The listing builds one solid part. Answer for the finished solid, in the listing's coordinates (mm). A direction names the side the tool comes from. Round coordinates to 2 decimals unless told otherwise and drop trailing zeros. Order: outer loops, then holes, each group sorted by start corner. A loop starts at its lowest first (then second) coordinate and runs counter-clockwise, first axis right, second up. Notation, with made-up numbers: (46.5, 51.25) - (105.5, 51.25) arc R26 cw to (105.5, 86.25) - close; hole circle Ø8 at (-7.75, -31.5). An arc over 180 degrees is marked (long way). One line per item, written item: value. Start each with the question number.
1. Section B-B, the plane z = -0.3 is taken. Give the vertices of the cut face in (x, y).
2. Section A-A, the plane y = -0.25 is taken. Give the vertices of the cut face in (x, z).
3. For a pull along X with two mould halves and no side action, classify faces 1 (the flat face through (3, 2, 0)), 2 (the flat face through (6.1, -3, -1.5)), 3 (the flat face through (3, 0, -2)), 4 (the flat face through (6.4, 0.5, -1.5)) as released by +X, released by -X, zero draft, split by the parting line, or undercut.
4. Section D-D, the plane y = 3.75 is taken. Give the vertices of the cut face in (x, z).
5. Flat-ended cylindrical pins translate along their axes: P1, Ø0.6, axis at y = 4, z = -1.5, coming from the +X side; P2, Ø0.5, axis at y = -3, z = -1.5, coming from the +X side; P3, Ø0.5, axis at y = -3, z = -1.5, coming from the -X side; P4, Ø2, axis at x = 1, y = -1.5, coming from the -Z side. Find the tip coordinate at first contact, or state that the pin passes through.
6. Section C-C, the plane x = 0.5 is taken. Give the vertices of the cut face in (y, z), then the cut area to 3 significant figures.
7. Straight lines are drawn through the part: line 1 (Y direction, x = 1.25, z = -2.8); line 2 (X direction, y = 3.25, z = -0.6); line 3 (X direction, y = -2.25, z = -1.75). For each, find the intervals that lie inside material, in ascending order.
8. A tool of negligible diameter and unlimited length cuts with its end or side. For faces 5 (the flat face through (3, 4.3, -2)), 6 (the flat face through (-0.4, 0.5, -1.5)), from which of +Z, -Z, +X, -X, +Y, -Y can it reach the whole face along a straight path? Write none if from no direction.
from build123d import *

# Parameters (mm, degrees)
SKETCH1_W           = 6
SKETCH1_H           = 3
BOSS_EXTRUDE1_DEPTH = 3.5
BOSS_EXTRUDE2_DEPTH = 0.5
SKETCH3_W           = 3
SKETCH3_H           = 1.5
BOSS_EXTRUDE3_DEPTH = 0.8
FILLET1_R           = 0.05


with BuildPart() as part:
    # Sketch1 → Boss-Extrude1 (new body)
    with BuildSketch(Plane(origin=(0, 0, 0), x_dir=(1, 0, 0), z_dir=(0, 1, 0))):
        with Locations((3, 1.5)):
            Rectangle(SKETCH1_W, SKETCH1_H)
    extrude(amount=BOSS_EXTRUDE1_DEPTH)

    # Sketch2 → Boss-Extrude2 (add, symmetric)
    with BuildSketch(Plane.XY.offset(-1.5)):
        Polygon((-0.1, 1.7), (0, 1.7), (0, 2), (-0.4, 2), (-0.4, -0.925735931), (-1.224264069, -1.75), (-0.4, -2.574264069), (-0.4, -3.5), (-0.1, -3.5), (-0.1, -2.45), (-0.8, -1.75), (-0.1, -1.05), (-0.1, -0.722730952), align=None)
    boss_extrude2 = extrude(amount=BOSS_EXTRUDE2_DEPTH, both=True)

    # Mirror1: Boss-Extrude2 across plane
    add(boss_extrude2.mirror(Plane.ZY.offset(-3)))

    # Sketch3 → Boss-Extrude3 (add)
    with BuildSketch(Plane(origin=(0, 3.5, 0), x_dir=(1, 0, 0), z_dir=(0, 1, 0))):
        with Locations((3, 1.5)):
            Rectangle(SKETCH3_W, SKETCH3_H)
    extrude(amount=BOSS_EXTRUDE3_DEPTH)

    # Fillet1
    fillet1_edges = [part.edges().sort_by_distance(p)[0] for p in [
        (6, 3.5, -1.5),
        (3, 3.5, -3),
        (-0.4, -3.5, -1.5),
        (-0.4, -3.037132034, -2),
        (-0.4, -2.574264069, -1.5),
        (-0.812132034, -2.162132034, -2),
        (-1.224264069, -1.75, -1.5),
        (-0.812132034, -1.337867966, -2),
        (-0.4, -0.925735931, -1.5),
        (-0.4, 0.537132034, -2),
        (-0.4, 2, -1.5),
        (0, 2, -1.5),
        (0, 1.85, -1),
        (0, 1.7, -1.5),
        (0, 1.85, -2),
        (-0.45, -2.1, -2),
        (-0.4, -3.037132034, -1),
        (-0.4, 0.537132034, -1),
        (-0.812132034, -1.337867966, -1),
        (-0.812132034, -2.162132034, -1),
        (0, 3.5, -1.5),
        (3, 0, -3),
        (6.4, -2.574264069, -1.5),
        (6.4, -3.037132034, -1),
        (6.4, -3.5, -1.5),
        (6.4, 2, -1.5),
        (6.4, 0.537132034, -1),
        (6, 0, -1.5),
        (6.4, -0.925735931, -1.5),
        (6.812132034, -1.337867966, -1),
        (7.224264069, -1.75, -1.5),
        (6.812132034, -2.162132034, -1),
        (6.4, -3.037132034, -2),
        (6.4, 0.537132034, -2),
        (6.812132034, -1.337867966, -2),
        (6.812132034, -2.162132034, -2),
        (3, 0, 0),
        (0, 0, -1.5),
        (3, 3.5, 0),
        (0, 1.75, -3),
        (4.5, 3.5, -1.5),
        (3, 3.5, -2.25),
        (6, 1.75, -3),
        (1.5, 3.5, -1.5),
        (3, 3.5, -0.75),
        (6, 1.75, 0),
        (4.5, 4.3, -1.5),
        (3, 4.3, -2.25),
        (1.5, 4.3, -1.5),
        (3, 4.3, -0.75),
        (0, 1.75, 0),
    ]]
    fillet(fillet1_edges, radius=FILLET1_R)


solid = part.part
Answer list:
1. outline: (0, 0.05) arc R0.05 ccw to (0.05, 0) - (5.95, 0) arc R0.05 ccw to (6, 0.05) - (6, 3.45) arc R0.05 ccw to (5.95, 3.5) - (0.05, 3.5) arc R0.05 ccw to (0, 3.45) - close
2. outline: (-0.4, -1.95) arc R0.05 ccw to (-0.35, -2) - (-0.1, -2) - (-0.1, -1) - (-0.35, -1) arc R0.05 ccw to (-0.4, -1.05) - close; (6.1, -2) - (6.35, -2) arc R0.05 ccw to (6.4, -1.95) - (6.4, -1.05) arc R0.05 ccw to (6.35, -1) - (6.1, -1) - close
3. face 1: zero draft
3. face 2: undercut
3. face 3: undercut
3. face 4: released by +X
4. outline: (1.5, -2.25) - (4.5, -2.25) - (4.5, -0.75) - (1.5, -0.75) - close
5. P1: stops at x = 4.5
5. P2: stops at x = 6.4
5. P3: stops at x = -0.4
5. P4: passes through
6. outline: (0, -2.95) arc R0.05 ccw to (0.05, -3) - (3.45, -3) arc R0.05 ccw to (3.5, -2.95) - (3.5, -0.05) arc R0.05 ccw to (3.45, 0) - (0.05, 0) arc R0.05 ccw to (0, -0.05) - close
6. area: 10.5 mm²
7. line 1: y = 0 to 3.5
7. line 2: x = 0 to 6
7. line 3: x = -0.72 to -0.3, 6.3 to 6.72
8. face 5: +Z, -Z, +X, -X, +Y
8. face 6: +Z, -Z, -X, +Y
